from build123d import *

# Parameters (mm, degrees)
SKETCH096_R      = 1
EXTRUDE013_DEPTH = 4
SKETCH095_R      = 1
EXTRUDE014_DEPTH = 4
SKETCH094_R      = 1
EXTRUDE012_DEPTH = 4
SKETCH093_W      = 10.5
SKETCH093_H      = 5.5
EXTRUDE011_DEPTH = 3.5


with BuildPart() as extrude013:
    # Sketch096 → Extrude013 (new body)
    with BuildSketch(Plane(origin=(8.25, 0.25, 0), x_dir=(1, 0, 0), z_dir=(0, 0, 1))):
        with Locations((1, 1)):
            Circle(SKETCH096_R)
        with Locations((1, 4)):
            Circle(SKETCH096_R)
    extrude(amount=EXTRUDE013_DEPTH)


with BuildPart() as extrude014:
    # Sketch095 → Extrude014 (new body)
    with BuildSketch(Plane(origin=(4.25, 0.25, 0), x_dir=(1, 0, 0), z_dir=(0, 0, 1))):
        with Locations((1, 1)):
            Circle(SKETCH095_R)
        with Locations((1, 4)):
            Circle(SKETCH095_R)
    extrude(amount=EXTRUDE014_DEPTH)


with BuildPart() as fusion008:
    # Sketch094 → Extrude012 (new body)
    with BuildSketch(Plane(origin=(0.25, 0.25, 0), x_dir=(1, 0, 0), z_dir=(0, 0, 1))):
        with Locations((1, 1)):
            Circle(SKETCH094_R)
        with Locations((1, 4)):
            Circle(SKETCH094_R)
    extrude(amount=EXTRUDE012_DEPTH)

    # Fusion008: union Extrude013, Extrude014
    add(extrude013.part)
    add(extrude014.part)


with BuildPart() as cut014:
    # Sketch093 → Extrude011 (new body)
    with BuildSketch(Plane.XY):
        with Locations((5.25, 2.75)):
            Rectangle(SKETCH093_W, SKETCH093_H)
    extrude(amount=EXTRUDE011_DEPTH)

    # Cut014: cut Fusion008
    add(fusion008.part, mode=Mode.SUBTRACT)


solid = cut014.part
Geometry: final body of the model. Coordinates: model frame, mm. Coordinates: 2 decimals unless noted, no trailing zeros. Order: outer loops, then holes, each group sorted by start corner. A loop starts at its lowest first (then second) coordinate and runs counter-clockwise, first axis right, second up. Notation, with made-up numbers: M 65.5,-22.5 L 112.5,-22.5 A29 ccw 112.5,4.5 Z; hole C 64,44.25 d2. An arc over 180 degrees is marked long. One line per question, with ' | ' between items. Start each with the question number.
Item 1: Ray query, probe 1 along X at (y, z) = (1.25, 2.1); probe 2 along Y at (x, z) = (1.25, 1.2); probe 3 along X at (y, z) = (3.4, 2.2). Return the intervals inside material, ascending. Write a range as [from, to].
Item 2: Cut plane A-A, the plane y = 1.25. Return the cut outline in (x, z).
Item 3: Draft query along Y for faces 1 (the flat face through (5, 3, 0)), 2 (the cylindrical face through (1.033, 0.274, 1.726)), 3 (the flat face through (5, 5.5, 2)). Return one class per face: released by +Y, released by -Y, zero draft, split by the parting line, or undercut.
Item 4: Cut plane D-D, the plane y = 0.45. Return the cut outline in (x, z), then the cut area to 4 significant figures.
Item 5: Cut plane B-B, the plane x = 1.25. Return the cut outline in (y, z), then the cut area to 3 significant figures.
Item 6: Cut plane C-C, the plane z = 1.1. Return the cut outline in (x, y).
A:
1) probe 1: x = [0, 0.25], [2.25, 4.25], [6.25, 8.25], [10.25, 10.5] | probe 2: y = [0, 0.25], [2.25, 3.25], [5.25, 5.5] | probe 3: x = [0, 0.72], [1.78, 4.72], [5.78, 8.72], [9.78, 10.5]
2) outline: M 0,0 L 0.25,0 L 0.25,3.5 L 0,3.5 Z; M 2.25,0 L 4.25,0 L 4.25,3.5 L 2.25,3.5 Z; M 6.25,0 L 8.25,0 L 8.25,3.5 L 6.25,3.5 Z; M 10.25,0 L 10.5,0 L 10.5,3.5 L 10.25,3.5 Z
3) face 1: zero draft | face 2: undercut | face 3: released by +Y
4) outline: M 0,0 L 0.65,0 L 0.65,3.5 L 0,3.5 Z; M 1.85,0 L 4.65,0 L 4.65,3.5 L 1.85,3.5 Z; M 5.85,0 L 8.65,0 L 8.65,3.5 L 5.85,3.5 Z; M 9.85,0 L 10.5,0 L 10.5,3.5 L 9.85,3.5 Z | area: 24.15 mm2
5) outline: M 0,0 L 0.25,0 L 0.25,3.5 L 0,3.5 Z; M 2.25,0 L 3.25,0 L 3.25,3.5 L 2.25,3.5 Z; M 5.25,0 L 5.5,0 L 5.5,3.5 L 5.25,3.5 Z | area: 5.25 mm2
6) outline: M 0,0 L 10.5,0 L 10.5,5.5 L 0,5.5 Z; hole C 1.25,1.25 d2; hole C 1.25,4.25 d2; hole C 5.25,1.25 d2; hole C 5.25,4.25 d2; hole C 9.25,1.25 d2; hole C 9.25,4.25 d2
